Read the model definition and answer for the solid it produces. Units are mm, in the model's axes. Coordinates: 2 decimals unless noted, no trailing zeros. Write each loop counter-clockwise with the first axis right and the second up, starting at its lowest first coordinate (ties: lowest second). Pieces come first, ordered by that corner, then holes. Notation, with made-up numbers: (49.5, 49.5) -> (77.5, 49.5) arc R23 cw to (77.5, 72.5) -> close; hole circle Ø7 at (28, 76.5). An arc over 180 degrees is marked (long way). Write item = value, one per line. Start each with the question number.
1) A flat-ended cylindrical pin translates along its axis: pin 1 Ø5.5 at (x, z) = (22.58, 4.64) entering from -Y. Find the tip coordinate at first contact, or state that the pin passes through.
2) For a pull along Z with two mould halves and no side action, classify faces 1 (the face through (24.96, -0.63, 5.38)), 2 (the face through (-15.395, -0.626, 27.422)), 3 (the face through (0, -1, 0)), 4 (the face through (-0.32, -0.63, 46.22)) as released by +Z, released by -Z, zero draft, split by the parting line, or undercut.
3) Section A-A (y = -0.55) is taken. Determine the outline of the cut face in (x, z), plus the area to 3 significant figures.
4) Find the intervals of material crossed by line 1 along X through (y, z) = (-0.35, 5.5); line 2 along X through (y, z) = (-1, 31.5); line 3 along X through (y, z) = (-0.15, 22.5), in increasing order. Write a range as from..to.
5) Section B-B (x = 14.5) is taken. Determine the outline of the cut face in (y, z).
6) Section C-C (z = 17.5) is taken. Determine the outline of the cut face in (x, y), plus the area to 3 significant figures.
from build123d import *

# Parameters (mm, degrees)
F0_R     = 2.49232
F1_DEPTH = 1.27


with BuildPart() as f1:
    # F0 (on Front) → F1 (new body)
    with BuildSketch(Plane.XZ):
        Polygon((0, 54.086622), (-31.226926, 0), (31.226926, 0), align=None)
        with Locations((-22.580516, 4.635875)):
            Circle(F0_R, mode=Mode.SUBTRACT)
        with Locations((22.580516, 4.635875)):
            Circle(F0_R, mode=Mode.SUBTRACT)
        with Locations((0, 43.746475)):
            Circle(F0_R, mode=Mode.SUBTRACT)
    extrude(amount=F1_DEPTH)


solid = f1.part
Answer key:
q1.pin_1 = -1.27
q2.face_1 = undercut
q2.face_2 = released by +Z
q2.face_3 = released by -Z
q2.face_4 = undercut
q3.outline = (-31.23, 0) -> (31.23, 0) -> (0, 54.09) -> close; hole circle Ø4.98 at (-22.58, 4.64); hole circle Ø4.98 at (0, 43.75); hole circle Ø4.98 at (22.58, 4.64)
q3.area = 1,630 mm^2
q4.line_1 = -28.05..-24.92, -20.24..20.24, 24.92..28.05
q4.line_2 = -13.04..13.04
q4.line_3 = -18.24..18.24
q5.outline = (-1.27, 0) -> (0, 0) -> (0, 28.97) -> (-1.27, 28.97) -> close
q6.outline = (-21.12, -1.27) -> (21.12, -1.27) -> (21.12, 0) -> (-21.12, 0) -> close
q6.area = 53.7 mm^2
